Autodesk Inventor part; units mm, degrees
ref_plane "YZ Plane" through (0, 0, 0) normal (1, 0, 0) x (0, 1, 0)
ref_plane "XZ Plane" through (0, 0, 0) normal (0, 1, 0) x (-1, 0, 0)
ref_plane "XY Plane" through (0, 0, 0) normal (0, 0, 1) x (1, 0, 0)
sketch "Sketch1" plane through (0, 0, 0) normal (0, 0, 1) x (1, 0, 0)
  circle A0 centre (-11.375, 11.375) radius 2.1
  circle A1 centre (-11.375, -11.375) radius 2.1
  line L0 (-15, 4.1) -> (-12.9, 4.1)
  line L1 (-12.9, 4.1) -> (-12.9, 8.28)
  line L2 (-12.9, 8.28) -> (-9.85, 8.28)
  line L3 (-9.85, 8.28) -> (-5.8, 4.23)
  line L4 (-5.8, 4.23) -> (-5.8, -4.23)
  line L5 (-5.8, -4.23) -> (-9.85, -8.28)
  line L6 (-9.85, -8.28) -> (-12.9, -8.28)
  line L7 (-12.9, -8.28) -> (-12.9, -4.1)
  line L8 (-12.9, -4.1) -> (-15, -4.1)
  line L9 (-15, -4.1) -> (-15, -13)
  arc A2 (-15, -13) -> (-13, -15) centre (-13, -13) ccw
  line L10 (-13, -15) -> (-4.1, -15)
  line L11 (-4.1, -15) -> (-4.1, -12.9)
  line L12 (-4.1, -12.9) -> (-8.28, -12.9)
  line L13 (-8.28, -12.9) -> (-8.28, -9.85)
  line L14 (-8.28, -9.85) -> (-3.719, -5.289)
  line L15 (-3.719, -5.289) -> (3.719, -5.289)
  line L16 (3.719, -5.289) -> (8.28, -9.85)
  line L17 (8.28, -9.85) -> (8.28, -12.9)
  line L18 (8.28, -12.9) -> (4.1, -12.9)
  line L19 (4.1, -12.9) -> (4.1, -15)
  line L20 (4.1, -15) -> (13, -15)
  arc A3 (13, -15) -> (15, -13) centre (13, -13) ccw
  line L21 (15, -13) -> (15, -4.1)
  line L22 (15, -4.1) -> (12.9, -4.1)
  line L23 (12.9, -4.1) -> (12.9, -8.28)
  line L24 (12.9, -8.28) -> (9.85, -8.28)
  line L25 (9.85, -8.28) -> (5.8, -4.23)
  line L26 (5.8, -4.23) -> (5.8, 4.23)
  line L27 (5.8, 4.23) -> (9.85, 8.28)
  line L28 (9.85, 8.28) -> (12.9, 8.28)
  line L29 (12.9, 8.28) -> (12.9, 4.1)
  line L30 (12.9, 4.1) -> (15, 4.1)
  line L31 (15, 4.1) -> (15, 13)
  arc A4 (15, 13) -> (13, 15) centre (13, 13) ccw
  line L32 (13, 15) -> (4.1, 15)
  line L33 (4.1, 15) -> (4.1, 12.9)
  line L34 (4.1, 12.9) -> (8.28, 12.9)
  line L35 (8.28, 12.9) -> (8.28, 9.85)
  line L36 (8.28, 9.85) -> (3.719, 5.289)
  line L37 (3.719, 5.289) -> (-3.719, 5.289)
  line L38 (-3.719, 5.289) -> (-8.28, 9.85)
  line L39 (-8.28, 9.85) -> (-8.28, 12.9)
  line L40 (-8.28, 12.9) -> (-4.1, 12.9)
  line L41 (-4.1, 12.9) -> (-4.1, 15)
  line L42 (-4.1, 15) -> (-13, 15)
  arc A5 (-13, 15) -> (-15, 13) centre (-13, 13) ccw
  line L43 (-15, 13) -> (-15, 4.1)
  circle A6 centre (0, 0) radius 3.4
  circle A7 centre (11.375, 11.375) radius 2.1
  circle A8 centre (11.375, -11.375) radius 2.1
extrude "Extrusion1" add sketch "Sketch1" against normal blind 500
properties part number "Metal Profile 50 cm" material "Aluminum 6061-AHC"
The listing builds one solid part. Answer for the finished solid, in the listing's coordinates (mm). Round coordinates to 2 decimals unless told otherwise and drop trailing zeros. Answer in a Markdown table with one row per item. Add a question column.
1) Flat-ended cylindrical pins translate along their axes: pin 1 Ø1 at (x, z) = (14, -328) entering from +Y; pin 2 Ø2.5 at (y, z) = (0, -296) entering from -X; pin 3 Ø0.6 at (y, z) = (14, -177) entering from -X. Find the tip coordinate at first contact, or state that the pin passes through.
2) Determine the mould class of faces 1 (the face through (9, 15, -246)), 2 (the face through (-15, 9, -246)), 3 (the face through (5.8, 0, -246)) for opening direction Y: pulls with the +Y half, pulls with the -Y half, needs draft (parallel to the pull), parting line crosses it, or undercut.
3) The part is cut by section A-A on z = -130.5. Count the separate pieces of the cut face and the enclosed holes in it, plus the area to 3 significant figures.
4) Consider line 1 along Y through (x, z) = (0, -125); line 2 along Y through (x, z) = (11.75, -228.5); line 3 along X through (y, z) = (-10.5, -371). Determine where each line is inside the solid, lowest interval first. Write a range as from..to.
Findings below:
| question | item | result |
|---|---|---|
| 1 | pin 1 | stops at y = 14.94 |
| 1 | pin 2 | stops at x = -5.8 |
| 1 | pin 3 | stops at x = -14.87 |
| 2 | face 1 | pulls with the +Y half |
| 2 | face 2 | needs draft |
| 2 | face 3 | undercut |
| 3 | separate pieces | 1 |
| 3 | enclosed holes | 5 |
| 3 | area | 323 mm² |
| 4 | line 1 | y = -5.29..-3.4, 3.4..5.29 |
| 4 | line 2 | y = -15..-13.44, -9.31..-8.28, 8.28..9.31, 13.44..15 |
| 4 | line 3 | x = -15..-13.28, -9.47..-8.28, 8.28..9.47, 13.28..15 |
